Part model, mm, in its own coordinate system. A direction names the side the tool comes from. Give positions to 0.01 mm unless a question says otherwise; leave off trailing zeros. Loops run counter-clockwise (first coordinate to the right, second up) from the corner with the lowest first, then second, coordinate; pieces in that order, holes last. Notation, with made-up numbers: (53, 18) -> (90, 18) arc R13 cw to (90, 34) -> close; hole circle Ø7 at (-36, 24.25). An arc over 180 degrees is marked (long way). One line per question, with ' | ' between items.
```python
from build123d import *

# Parameters (mm, degrees)
SKETCH_1_W          = 20
SKETCH_1_H          = 26.5
SKETCH_1_R          = 2
EXTRUDE_1_DEPTH     = 3
SKETCH_2_W          = 20
SKETCH_2_H          = 3
EXTRUDE_2_DEPTH     = 24
EXTRUDE_3_DEPTH     = 2
SKETCH_5_W          = 12.5
SKETCH_5_H          = 3.5
EXTRUDE_4_DEPTH     = 20
SKETCH_4_R          = 1.5
CUT_EXTRUDE_1_DEPTH = 10
FILLET_1_R          = 10


with BuildPart() as part:
    # 草图1 → 凸台-拉伸1 (new body)
    with BuildSketch(Plane.XY):
        with Locations((10, -41.75)):
            Rectangle(SKETCH_1_W, SKETCH_1_H)
        with Locations((5, -45.291502622)):
            Circle(SKETCH_1_R, mode=Mode.SUBTRACT)
        with Locations((15, -45.291502622)):
            Circle(SKETCH_1_R, mode=Mode.SUBTRACT)
    extrude(amount=EXTRUDE_1_DEPTH)

    # 草图2 → 凸台-拉伸2 (add)
    with BuildSketch(Plane.XY):
        with Locations((10, -30)):
            Rectangle(SKETCH_2_W, SKETCH_2_H)
    extrude(amount=-EXTRUDE_2_DEPTH)

    # 草图3 → 凸台-拉伸3 (add)
    with BuildSketch(Plane(origin=(0, 0, 0), x_dir=(0, 0, -1), z_dir=(1, 0, 0))):
        Polygon((0, -31.5), (0, -42.5), (15, -31.5), align=None)
    extrude_3 = extrude(amount=EXTRUDE_3_DEPTH)

    # 镜向1: 凸台-拉伸3 across plane
    add(extrude_3.mirror(Plane(origin=(10, 0, 0), x_dir=(0, 0, 1), z_dir=(1, 0, 0))))

    # 草图5 → 凸台-拉伸4 (add)
    with BuildSketch(Plane(origin=(0, 0, 0), x_dir=(0, 0, -1), z_dir=(1, 0, 0))):
        with Locations((17.75, -26.75)):
            Rectangle(SKETCH_5_W, SKETCH_5_H)
    extrude(amount=EXTRUDE_4_DEPTH)

    # 草图4 → 切除-拉伸1 (cut, symmetric)
    with BuildSketch(Plane(origin=(0, -28.5, 0), x_dir=(1, 0, 0), z_dir=(0, 1, 0))):
        with Locations(Location((10, 20, 0), (0, 0, 270))):
            Circle(SKETCH_4_R)
    extrude(amount=CUT_EXTRUDE_1_DEPTH, both=True, mode=Mode.SUBTRACT)

    # 圆角1
    # the kernel refuses this fillet: 10 mm, written as the material it adds along each edge
    with BuildSketch(Plane(origin=(0, -28.5, -11.5), x_dir=(0, 0, 1), z_dir=(1, 0, 0))) as fillet_1_piece_1:
        with BuildLine():
            CenterArc((7.599342077, -10), FILLET_1_R, 90, 49.458398126)
            Line((0, -3.5), (-0.151986842, -3.37))
            ThreePointArc((-0.151986842, -3.37), (-0.2, -1.75), (-0.2, 0))
            Line((-0.2, 0), (0, 0.2))
            Line((0, 0.2), (7.599342077, 0.2))
            Line((7.599342077, 0.2), (7.599342077, 0))
        make_face()
    extrude(amount=20)


solid = part.part
```
1) Saw through at B-B (z = -20). Give the cut face in (x, y), and give its area (4 significant figures).
Found:
outline: (0, -31.5) -> (8.5, -31.5) -> (8.5, -25) -> (0, -25) -> close; (11.5, -31.5) -> (20, -31.5) -> (20, -25) -> (11.5, -25) -> close | area: 110.5 mm2
2) Saw through at D-D (x = 10). Give the cut face in (y, z), and give its area (3 significant figures).
Found:
outline: (-55, 0) -> (-31.5, 0) -> (-31.5, -18.5) -> (-25, -18.5) -> (-25, -11.5) arc R10 cw to (-28.5, -3.9) -> (-28.5, 3) -> (-55, 3) -> close; (-31.5, -24) -> (-25, -24) -> (-25, -21.5) -> (-31.5, -21.5) -> close | area: 184 mm2
3) Saw through at A-A (x = 15). Give the cut face in (y, z).
Found:
outline: (-55, 0) -> (-47.29, 0) -> (-47.29, 3) -> (-55, 3) -> close; (-43.29, 0) -> (-31.5, 0) -> (-31.5, -24) -> (-25, -24) -> (-25, -11.5) arc R10 cw to (-28.5, -3.9) -> (-28.5, 3) -> (-43.29, 3) -> close
4) Pull direction X, two halves, no side cores. Call faces 1 (the flat face through (2, -36, -6)), 2 (the flat face through (0.986, -37.077, -7.395)), 3 (the flat face through (0, -35, -7)): pulls with the +X half, pulls with the -X half, needs draft (parallel to the pull), parting line crosses it, or undercut.
Found:
face 1: undercut | face 2: needs draft | face 3: pulls with the -X half
5) Saw through at C-C (y = -40.5). Give the cut face in (x, z).
Found:
outline: (0, -2.73) -> (2, -2.73) -> (2, 0) -> (18, 0) -> (18, -2.73) -> (20, -2.73) -> (20, 3) -> (0, 3) -> close
6) Tool access for faces 4 (the flat face through (10, -31.5, -12)), 5 (the flat face through (10, -42, 3)), 6 (the flat face through (10, -28.5, 0)): list every direction of +Z, -Z, +X, -X, +Y, -Y with a clear straight run to the whole face (end or side of a thin tool).
Found:
face 4: -Z, -Y | face 5: +Z, +X, -X, +Y, -Y | face 6: +Z, +X, -X, +Y
7) Pin check, flat tips, straight feed: P1, Ø7.5, axis at x = 9, z = -0.5, coming from the +Y side; P2, Ø6, axis at x = 6, y = -45.5, coming from the -Z side; P3, Ø8, axis at x = 16.5, z = -4.5, coming from the +Y side; P4, Ø3, axis at x = 5, y = -45.29, coming from the -Z side. Stop position of each tip, or through.
Found:
P1: y = -28.49 | P2: z = 0 | P3: y = -27.38 | P4: through
8) Drill centre lines: line 1 (Y direction, x = 5, z = 2.25); line 2 (X direction, y = -28.75, z = -20); line 3 (Y direction, x = 4, z = -0.25). Where is each one in solid material? Low to high.
Found:
line 1: -55 to -47.29, -43.29 to -28.5 | line 2: 0 to 8.5, 11.5 to 20 | line 3: -31.5 to -28.5
